from build123d import *

# Parameters (mm, degrees)
F0_W     = 203.2
F0_H     = 127
F1_DEPTH = 6.35
F3_DEPTH = 6.35


with BuildPart() as f1:
    # F0 (on Front) → F1 (new body)
    with BuildSketch(Plane.XZ):
        Rectangle(F0_W, F0_H)
    extrude(amount=F1_DEPTH)

    # F2 (on face) → F3 (cut, through all)
    with BuildSketch(Plane.XZ.offset(6.35)):
        with BuildLine():
            Line((-68.072, 9.017), (-68.072, 0))
            Line((-68.072, 0), (-68.072, -9.017))
            ThreePointArc((-68.072, -9.017), (-57.15, -14.276614), (-46.228, -9.017))
            Line((-46.228, -9.017), (-46.228, 0))
            Line((-46.228, 0), (-46.228, 9.017))
            ThreePointArc((-46.228, 9.017), (-57.15, 14.276614), (-68.072, 9.017))
        make_face()
        with BuildLine():
            Line((-29.972, 9.017), (-29.972, 0))
            Line((-29.972, 0), (-29.972, -9.017))
            ThreePointArc((-29.972, -9.017), (-19.05, -14.276614), (-8.128, -9.017))
            Line((-8.128, -9.017), (-8.128, 0))
            Line((-8.128, 0), (-8.128, 9.017))
            ThreePointArc((-8.128, 9.017), (-19.05, 14.276614), (-29.972, 9.017))
        make_face()
        with BuildLine():
            Line((8.128, 9.017), (8.128, 0))
            Line((8.128, 0), (8.128, -9.017))
            ThreePointArc((8.128, -9.017), (19.05, -14.276614), (29.972, -9.017))
            Line((29.972, -9.017), (29.972, 0))
            Line((29.972, 0), (29.972, 9.017))
            ThreePointArc((29.972, 9.017), (19.05, 14.276614), (8.128, 9.017))
        make_face()
        with BuildLine():
            Line((46.228, 9.017), (46.228, 0))
            Line((46.228, 0), (46.228, -9.017))
            ThreePointArc((46.228, -9.017), (57.15, -14.276614), (68.072, -9.017))
            Line((68.072, -9.017), (68.072, 0))
            Line((68.072, 0), (68.072, 9.017))
            ThreePointArc((68.072, 9.017), (57.15, 14.276614), (46.228, 9.017))
        make_face()
    extrude(amount=-F3_DEPTH, mode=Mode.SUBTRACT)


solid = f1.part
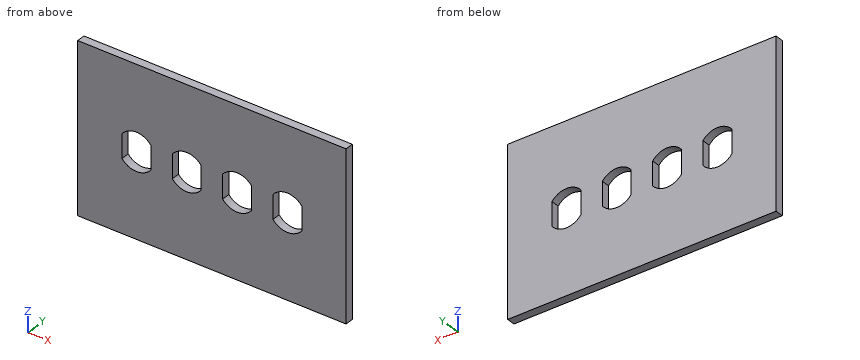
CAD build for the part. Positions are in the model's coordinates, mm. Give positions to 0.01 mm unless a question says otherwise; leave off trailing zeros. Order: outer loops, then holes, each group sorted by start corner. A loop starts at its lowest first (then second) coordinate and runs counter-clockwise, first axis right, second up. Notation, with made-up numbers: (83.5, 29.5) - (128.5, 29.5) arc R24 ccw to (128.5, 48.5) - close; hole circle Ø4 at (-34.5, 67). An arc over 180 degrees is marked (long way). Answer in a Markdown table with one row per item.
1. Saw through at B-B, the plane x = -50. Give the cut face in (y, z), plus the area to 3 significant figures.
Data:
| item | result |
|---|---|
| outline | (-6.35, -63.5) - (0, -63.5) - (0, -12.31) - (-6.35, -12.31) - close; (-6.35, 12.31) - (0, 12.31) - (0, 63.5) - (-6.35, 63.5) - close |
| area | 650 mm² |
2. Probe probe 1 along X at (y, z) = (-0.75, 2); probe 2 along X at (y, z) = (-1, 11); probe 3 along Z at (x, y) = (-58, -0.75). List the from-to ranges inside material, lowest first. Write a range as [from, to].
Data:
| item | result |
|---|---|
| probe 1 | x = [-101.6, -68.07], [-46.23, -29.97], [-8.13, 8.13], [29.97, 46.23], [68.07, 101.6] |
| probe 2 | x = [-101.6, -66.14], [-48.16, -28.04], [-10.06, 10.06], [28.04, 48.16], [66.14, 101.6] |
| probe 3 | z = [-63.5, -14.25], [14.25, 63.5] |
3. Saw through at D-D, the plane x = 12. Give the cut face in (y, z).
Data:
| item | result |
|---|---|
| outline | (-6.35, -63.5) - (0, -63.5) - (0, -12.37) - (-6.35, -12.37) - close; (-6.35, 12.37) - (0, 12.37) - (0, 63.5) - (-6.35, 63.5) - close |
4. Saw through at A-A, the plane y = -5.25. Give the cut face in (x, z), plus the area to 3 significant figures.
Data:
| item | result |
|---|---|
| outline | (-101.6, -63.5) - (101.6, -63.5) - (101.6, 63.5) - (-101.6, 63.5) - close; hole (-68.07, -9.02) arc R13.97 ccw to (-46.23, -9.02) - (-46.23, 9.02) arc R13.97 ccw to (-68.07, 9.02) - close; hole (-29.97, -9.02) arc R13.97 ccw to (-8.13, -9.02) - (-8.13, 9.02) arc R13.97 ccw to (-29.97, 9.02) - close; hole (8.13, -9.02) arc R13.97 ccw to (29.97, -9.02) - (29.97, 9.02) arc R13.97 ccw to (8.13, 9.02) - close; hole (46.23, -9.02) arc R13.97 ccw to (68.07, -9.02) - (68.07, 9.02) arc R13.97 ccw to (46.23, 9.02) - close |
| area | 23,600 mm² |
5. Saw through at C-C, the plane z = 12. Give the cut face in (x, y).
Data:
| item | result |
|---|---|
| outline | (-101.6, -6.35) - (-64.79, -6.35) - (-64.79, 0) - (-101.6, 0) - close; (-49.51, -6.35) - (-26.69, -6.35) - (-26.69, 0) - (-49.51, 0) - close; (-11.41, -6.35) - (11.41, -6.35) - (11.41, 0) - (-11.41, 0) - close; (26.69, -6.35) - (49.51, -6.35) - (49.51, 0) - (26.69, 0) - close; (64.79, -6.35) - (101.6, -6.35) - (101.6, 0) - (64.79, 0) - close |
